```python
from build123d import *

# Parameters (mm, degrees)
PAD_DEPTH = 0.9
FILLET_R  = 0.6


with BuildPart() as part:
    # Sketch → Pad (new body)
    with BuildSketch(Plane.XY):
        with BuildLine():
            ThreePointArc((3.749388, -4.684238), (0, 6), (-3.749388, -4.684238))
            Line((-2.75, -1.198958), (-3.749388, -4.684238))
            ThreePointArc((-2.85317, 0.927051), (-2.996474, -0.145411), (-2.75, -1.198958))
            Line((-2.85317, 0.927051), (-4.279754, 1.390576))
            ThreePointArc((-1.390576, 4.279754), (-3.181981, 3.181981), (-4.279754, 1.390576))
            Line((-0.927051, 2.85317), (-1.390576, 4.279754))
            ThreePointArc((0.927051, 2.85317), (0, 3), (-0.927051, 2.85317))
            Line((0.927051, 2.85317), (1.390576, 4.279754))
            ThreePointArc((4.279754, 1.390576), (3.181981, 3.181981), (1.390576, 4.279754))
            Line((4.279754, 1.390576), (2.85317, 0.927051))
            ThreePointArc((2.75, -1.198958), (2.996474, -0.145411), (2.85317, 0.927051))
            Line((2.75, -1.198958), (3.749388, -4.684238))
        make_face()
    extrude(amount=PAD_DEPTH)

    # Fillet
    fillet_edges = [part.edges().sort_by_distance(p)[0] for p in [
        (3.749388, -4.684238, 0.45),
        (2.75, -1.198958, 0.45),
        (2.85317, 0.927051, 0.45),
        (4.279754, 1.390576, 0.45),
        (1.390576, 4.279754, 0.45),
        (0.927051, 2.85317, 0.45),
        (-0.927051, 2.85317, 0.45),
        (-1.390576, 4.279754, 0.45),
        (-4.279754, 1.390576, 0.45),
        (-2.85317, 0.927051, 0.45),
        (-2.75, -1.198958, 0.45),
        (-3.749388, -4.684238, 0.45),
    ]]
    fillet(fillet_edges, radius=FILLET_R)


solid = part.part
```
Input: part model. Units: mm. Frame: model coordinates. A direction names the side the tool comes from. Coordinates: 2 decimals unless noted, no trailing zeros. Loops run counter-clockwise (first coordinate to the right, second up) from the corner with the lowest first, then second, coordinate; pieces in that order, holes last.
Q1. Section D-D, the plane y = 0.75. Return the cut outline in (x, z).
Results are:
outline: (-5.95, 0) - (-3, 0) - (-3, 0.9) - (-5.95, 0.9) - close; (3, 0) - (5.95, 0) - (5.95, 0.9) - (3, 0.9) - close
Q2. Mould query, pull axis X, two halves, no side actions, for faces 4 (the cylindrical face through (0.193, 5.997, 0.444)), 5 (the cylindrical face through (0, 3, 0.4)), 6 (the flat face through (-0.1, 3.2, 0.9)). Classes: +X half, -X half, draft (parallel to the pull), parting line (faces both ways), or undercut.
Results are:
face 4: parting line
face 5: undercut
face 6: draft
Q3. Set-up query: faces 1 (the flat face through (3.137, -2.548, 0.444)), 2 (the flat face through (-0.1, 3.2, 0)), 3 (the cylindrical face through (3.196, 3.168, 0.444)). Return all of +Z, -Z, +X, -X, +Y, -Y with unobstructed straight access to the full face (end or side cutting, diameter ignored); none if empty.
Results are:
face 1: +Z, -Z, -Y
face 2: -Z, +X, -X, +Y, -Y
face 3: +Z, -Z
Q4. Section B-B, the plane z = 0.5. Return the cut outline in (x, y).
Results are:
outline: (-4.5, -3.96) arc R0.6 ccw to (-3.48, -3.73) - (-2.81, -1.4) arc R0.6 ccw to (-2.82, -1.03) arc R3 cw to (-2.97, 0.44) arc R0.6 ccw to (-3.38, 1.1) - (-3.66, 1.19) arc R0.6 cw to (-4.01, 2.03) arc R4.5 cw to (-2.03, 4.01) arc R0.6 cw to (-1.19, 3.66) - (-1.1, 3.38) arc R0.6 ccw to (-0.44, 2.97) arc R3 cw to (0.44, 2.97) arc R0.6 ccw to (1.1, 3.38) - (1.19, 3.66) arc R0.6 cw to (2.03, 4.01) arc R4.5 cw to (4.01, 2.03) arc R0.6 cw to (3.66, 1.19) - (3.38, 1.1) arc R0.6 ccw to (2.97, 0.44) arc R3 cw to (2.82, -1.03) arc R0.6 ccw to (2.81, -1.4) - (3.48, -3.73) arc R0.6 ccw to (4.5, -3.96) arc R6 ccw (long way) to start
Q5. Section A-A, the plane y = -0.5. Return the cut outline in (x, z), and give its area (3 significant figures).
Results are:
outline: (-5.98, 0) - (-2.96, 0) - (-2.96, 0.9) - (-5.98, 0.9) - close; (2.96, 0) - (5.98, 0) - (5.98, 0.9) - (2.96, 0.9) - close
area: 5.44 mm2
Q6. Section C-C, the plane x = 0. Return the cut outline in (y, z), and give its area (3 significant figures).
Results are:
outline: (3, 0) - (6, 0) - (6, 0.9) - (3, 0.9) - close
area: 2.70 mm2
Q7. Line query: line 1 along X through (y, z) = (3.75, 0.25); line 2 along X through (y, z) = (3.25, 0.55); line 3 along X through (y, z) = (0, 0.55). Output: solid intervals per line, ascending.
Results are:
line 1: x = -4.68 to -2.49, -1.23 to 1.23, 2.49 to 4.68
line 2: x = -5.04 to -3.11, -1.04 to 1.04, 3.11 to 5.04
line 3: x = -6 to -3, 3 to 6
